Could you check a few things on this model? Use its own coordinates, in mm. Coordinates: 2 decimals unless noted, no trailing zeros. Order: outer loops, then holes, each group sorted by start corner. A loop starts at its lowest first (then second) coordinate and runs counter-clockwise, first axis right, second up. Notation, with made-up numbers: (82.5, 75) - (125.5, 75) arc R8 cw to (125.5, 87) - close; hole circle Ø2 at (-3.75, 22). An arc over 180 degrees is marked (long way). Answer as a JSON object with one key per item and string values. Group by question number.
(1) Please list where these lines run through material, in increasing order: probe 1 along X at (y, z) = (14, -18.5); probe 2 along X at (y, z) = (-21, 1); probe 3 along X at (y, z) = (177, 9).
(2) Imagine slicing it at D-D, the plane x = 850. Write out the boundary of the cut face in (y, z).
(3) Imagine slicing it at B-B, the plane y = 81.5. Write out the boundary of the cut face in (x, z), and give its area (3 significant figures).
(4) Will these pins go through, and if not, where does the flat tip stop? P1, Ø6, axis at y = 9, z = 17.5, coming from the -X side; P2, Ø22, axis at y = 42, z = -6.5, coming from the -X side; P3, Ø16, axis at y = -8, z = 13.5, coming from the -X side.
(5) Imagine slicing it at C-C, the plane y = 0. Write out the boundary of the cut face in (x, z).
(6) Imagine slicing it at A-A, the plane x = -550. Write out the boundary of the cut face in (y, z).
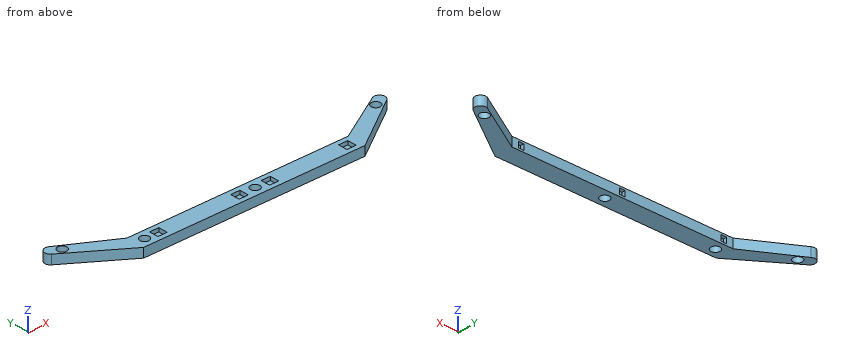
from build123d import *

# Parameters (mm, degrees)
BOSS_EXTRUDE1_DEPTH      = 600
BOSS_EXTRUDE1_DEPTH_BACK = 600
SKETCH1_W                = 50
SKETCH1_H                = 100
BOSS_EXTRUDE2_DEPTH      = 50
SKETCH3_R                = 25
CUT_EXTRUDE1_DEPTH       = 50
SKETCH4_R                = 25
CUT_EXTRUDE2_DEPTH       = 948.9580797
SKETCH5_W                = 50
SKETCH5_H                = 50
CUT_EXTRUDE3_DEPTH       = 20
SKETCH6_W                = 30
SKETCH6_H                = 30
CUT_EXTRUDE4_DEPTH       = 20


with BuildPart() as part:
    # Sketch1 → Boss-Extrude1 (new, two sides: drawn at the far end of the back side and taken through both)
    with BuildSketch(Plane(origin=(0, 0, 0), x_dir=(0, 0, -1), z_dir=(1, 0, 0)).offset(-BOSS_EXTRUDE1_DEPTH_BACK)):
        Rectangle(SKETCH1_W, SKETCH1_H)
    extrude(amount=BOSS_EXTRUDE1_DEPTH + BOSS_EXTRUDE1_DEPTH_BACK)

    # Sketch2 → Boss-Extrude2 (add)
    with BuildSketch(Plane.XY.offset(25)):
        with BuildLine():
            Line((600, 50), (877.128129211, 210))
            ThreePointArc((877.128129211, 210), (917.555611759, 199.939135225), (908.947540593, 159.177591388))
            Line((908.947540593, 159.177591388), (600, -50))
            Line((600, -50), (600, 50))
        make_face()
        with BuildLine():
            Line((-600, 50), (-600, -50))
            Line((-600, -50), (-908.947540593, 159.177591388))
            ThreePointArc((-908.947540593, 159.177591388), (-917.555611759, 199.939135225), (-877.128129211, 210))
            Line((-877.128129211, 210), (-600, 50))
        make_face()
    extrude(amount=-BOSS_EXTRUDE2_DEPTH)

    # Sketch3 → Cut-Extrude1 (cut)
    with BuildSketch(Plane.XY.offset(25)):
        with Locations((-850, 160)):
            Circle(SKETCH3_R)
        with Locations(Location((850, 160, 0), (0, 0, 180))):
            Circle(SKETCH3_R)
    extrude(amount=-CUT_EXTRUDE1_DEPTH, mode=Mode.SUBTRACT)

    # Sketch4 → Cut-Extrude2 (cut, through all)
    with BuildSketch(Plane.XY.offset(25)):
        with Locations((50, 0)):
            Circle(SKETCH4_R)
        with Locations((-550, 0)):
            Circle(SKETCH4_R)
    extrude(amount=-CUT_EXTRUDE2_DEPTH, mode=Mode.SUBTRACT)

    # Sketch5 → Cut-Extrude3 (cut)
    with BuildSketch(Plane.XY.offset(25)):
        with Locations((-35, 0)):
            Rectangle(SKETCH5_W, SKETCH5_H)
        with Locations((-475, 0)):
            Rectangle(SKETCH5_W, SKETCH5_H)
        with Locations((130, 0)):
            Rectangle(SKETCH5_W, SKETCH5_H)
        with Locations((550, 0)):
            Rectangle(SKETCH5_W, SKETCH5_H)
    extrude(amount=-CUT_EXTRUDE3_DEPTH, mode=Mode.SUBTRACT)

    # Sketch6 → Cut-Extrude4 (cut)
    with BuildSketch(Plane(origin=(0, 50, 0), x_dir=(1, 0, 0), z_dir=(0, 1, 0))):
        with Locations((550, 0)):
            Rectangle(SKETCH6_W, SKETCH6_H)
        with Locations((-550, 0)):
            Rectangle(SKETCH6_W, SKETCH6_H)
        Rectangle(SKETCH6_W, SKETCH6_H)
    extrude(amount=-CUT_EXTRUDE4_DEPTH, mode=Mode.SUBTRACT)


solid = part.part
Result set:
{
 "1": {"probe 1": "x = -694.53 to -570.71, -529.29 to 29.29, 70.71 to 694.53", "probe 2": "x = -642.83 to -563.56, -536.44 to 36.44, 63.56 to 642.83", "probe 3": "x = -921.3 to -868.33, -831.67 to -819.97, 819.97 to 831.67, 868.33 to 921.3"},
 "2": {"outline": "(119.27, -25) - (135, -25) - (135, 25) - (119.27, 25) - close; (185, -25) - (194.34, -25) - (194.34, 25) - (185, 25) - close"},
 "3": {"outline": "(-794.22, -25) - (-654.56, -25) - (-654.56, 25) - (-794.22, 25) - close; (654.56, -25) - (794.22, -25) - (794.22, 25) - (654.56, 25) - close", "area": "14,000 mm^2"},
 "4": {"P1": "stops at x = -691.57", "P2": "stops at x = -752.13", "P3": "stops at x = -673.85"},
 "5": {"outline": "(-673.85, -25) - (-575, -25) - (-575, 25) - (-673.85, 25) - close; (-525, -25) - (25, -25) - (25, 25) - (-10, 25) - (-10, 5) - (-60, 5) - (-60, 25) - (-450, 25) - (-450, 5) - (-500, 5) - (-500, 25) - (-525, 25) - close; (75, -25) - (673.85, -25) - (673.85, 25) - (575, 25) - (575, 5) - (525, 5) - (525, 25) - (155, 25) - (155, 5) - (105, 5) - (105, 25) - (75, 25) - close"},
 "6": {"outline": "(-50, -25) - (-25, -25) - (-25, 25) - (-50, 25) - close; (25, -25) - (50, -25) - (50, -15) - (30, -15) - (30, 15) - (50, 15) - (50, 25) - (25, 25) - close"}
}
